Print and shaded views of the part. All mm, measured from the part's lowest x, y and z. Coordinates: 2 decimals unless noted, no trailing zeros. Write each loop counter-clockwise with the first axis right and the second up, starting at its lowest first coordinate (ties: lowest second). Pieces come first, ordered by that corner, then holes. Notation, with made-up numbers: (15, 86) -> (28, 86) arc R28 cw to (28, 113) -> close; hole circle Ø2 at (-16.75, -38). An arc over 180 degrees is marked (long way). Write item = value, one per line.
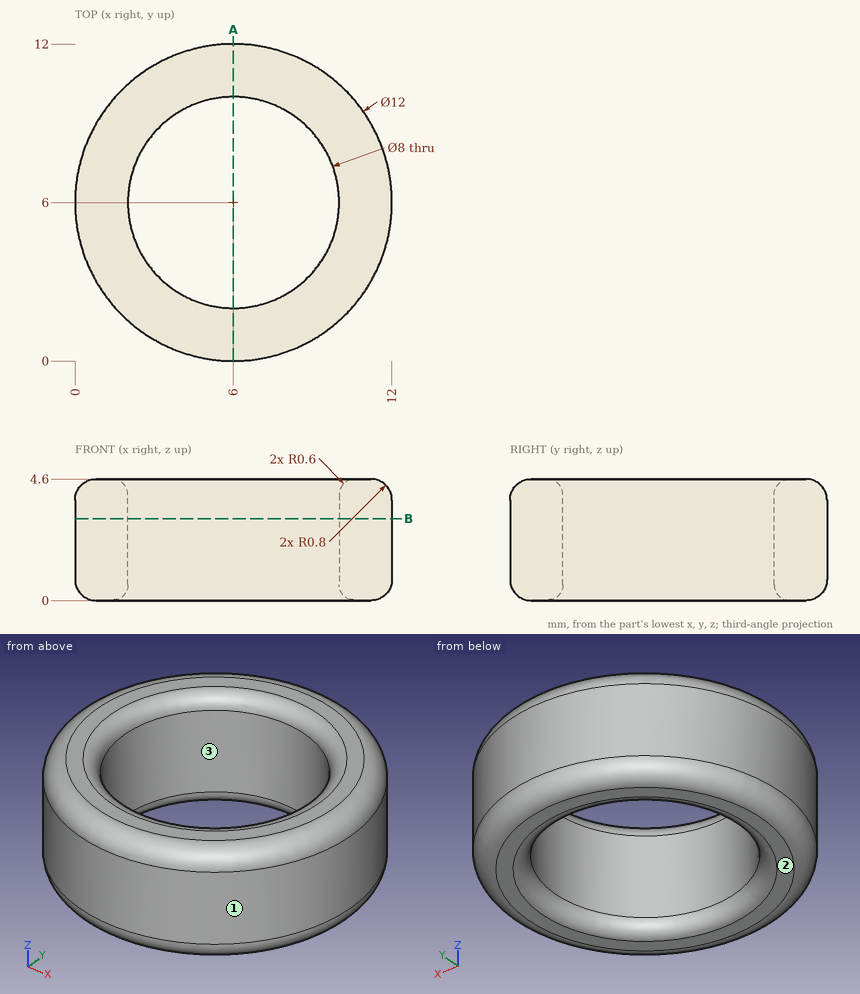
Q1. Saw through at B-B on z = 3.1. Give the cut face in (x, y), and give its area (3 significant figures).
Model answer:
outline = circle Ø12 at (6, 6); hole circle Ø8 at (6, 6)
area = 62.8 mm²
Q2. Probe line 1 (Y direction, x = 6, z = 2.7); line 2 (Y direction, x = 8.5, z = 4.3); line 3 (Z direction, x = 1.5, y = 8.75). List the from-to ranges inside material, lowest first. Write a range as from..to.
Model answer:
line_1 = 0..2, 10..12
line_2 = 0.74..2.78, 9.22..11.26
line_3 = 0..4.6
Q3. Saw through at A-A on x = 6. Give the cut face in (y, z).
Model answer:
outline = (0, 0.8) arc R0.8 ccw to (0.8, 0) -> (1.4, 0) arc R0.6 ccw to (2, 0.6) -> (2, 4) arc R0.6 ccw to (1.4, 4.6) -> (0.8, 4.6) arc R0.8 ccw to (0, 3.8) -> close; (10, 0.6) arc R0.6 ccw to (10.6, 0) -> (11.2, 0) arc R0.8 ccw to (12, 0.8) -> (12, 3.8) arc R0.8 ccw to (11.2, 4.6) -> (10.6, 4.6) arc R0.6 ccw to (10, 4) -> close
Q4. Mould opens along X. For the marked faces 1, 2 and 3 say: released by +X, released by -X, zero draft, split by the parting line, or undercut.
Model answer:
face_1 = split by the parting line
face_2 = zero draft
face_3 = undercut
Q5. Pin check, flat tips, straight feed: pin 1 (2 mm diameter, centred on y = 4.5, z = 2.5, fed in from +X); pin 2 (5 mm diameter, centred on x = 6, y = 6, fed in from +Z); pin 3 (1 mm diameter, centred on y = 4.5, z = 4, fed in from -X); pin 4 (4 mm diameter, centred on x = 8, y = 5, fed in from +Z). Stop position of each tip, or through.
Model answer:
pin_1 = 11.98
pin_2 = through
pin_3 = 0.09
pin_4 = 4.48
